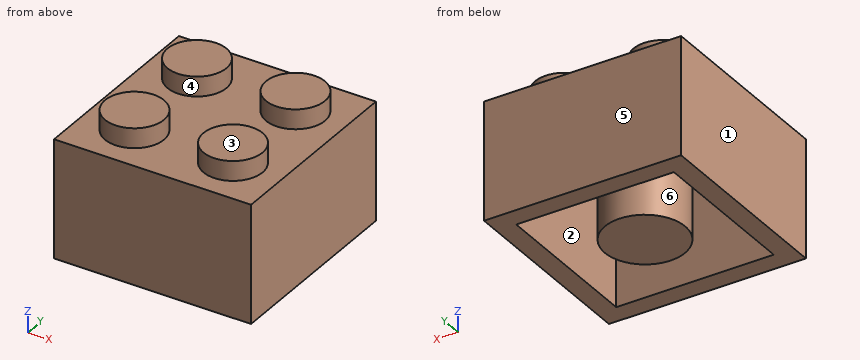
from build123d import *

# Parameters (mm, degrees)
F0_W     = 16
F0_H     = 16
F1_DEPTH = 9.6
F2_W     = 12.8
F2_H     = 12.8
F2_R     = 3.2565
F3_DEPTH = 8
F4_R     = 2.4
F5_DEPTH = 1.6
F6_R     = 1.2
F7_DEPTH = 1.6


with BuildPart() as f1:
    # F0 (on Top) → F1 (new body)
    with BuildSketch(Plane.XY):
        Rectangle(F0_W, F0_H)
    extrude(amount=F1_DEPTH)

    # F2 (on face) → F3 (cut)
    with BuildSketch(Plane(origin=(0, 0, 0), x_dir=(1, 0, 0), z_dir=(0, 0, -1))):
        Rectangle(F2_W, F2_H)
        Circle(F2_R, mode=Mode.SUBTRACT)
    extrude(amount=-F3_DEPTH, mode=Mode.SUBTRACT)

    # F4 (on face) → F5 (join)
    with BuildSketch(Plane.XY.offset(9.6)):
        with Locations((-4, 4)):
            Circle(F4_R)
        with Locations((4, 4)):
            Circle(F4_R)
        with Locations((-4, -4)):
            Circle(F4_R)
        with Locations((4, -4)):
            Circle(F4_R)
    extrude(amount=F5_DEPTH)

    # F6 (on face) → F7 (cut)
    with BuildSketch(Plane(origin=(0, 0, 8), x_dir=(1, 0, 0), z_dir=(0, 0, -1))):
        with Locations((-4, -4)):
            Circle(F6_R)
        with Locations((4, -4)):
            Circle(F6_R)
        with Locations((-4, 4)):
            Circle(F6_R)
        with Locations((4, 4)):
            Circle(F6_R)
    extrude(amount=-F7_DEPTH, mode=Mode.SUBTRACT)


solid = f1.part
Here's how the part is built. I have some questions about the finished solid (model axes, mm). Face numbers are marked on the shaded views. A direction names the side the tool comes from. Round coordinates to 2 decimals unless told otherwise and drop trailing zeros. Loops run counter-clockwise (first coordinate to the right, second up) from the corner with the lowest first, then second, coordinate; pieces in that order, holes last. Notation, with made-up numbers: (87, 77.25) -> (122, 77.25) arc R18 cw to (122, 106.25) -> close; hole circle Ø11 at (69.5, 66). An arc over 180 degrees is marked (long way). Write each question's results on one line, items separated by ' | '.
(1) For the marked faces 4, 5 and 6, which set-ups out of +Z, -Z, +X, -X, +Y, -Y let a thin tool reach every point of the face, with its end or its side?
Worked answers:
face 4: +Z | face 5: +Z, -Z, +X, -X, +Y | face 6: -Z
(2) If I drill on L1, parallel to X at y = 4, z = 8.75; L2, parallel to X at y = 0, z = 4, over which ranges is the centre line in solid material (lowest first)?
Worked answers:
L1: -8 to -5.2, -2.8 to 2.8, 5.2 to 8 | L2: -8 to -6.4, -3.26 to 3.26, 6.4 to 8
(3) For P1, Ø3, axis at x = 2, y = -2, coming from the +Z side; P2, Ø1.2, axis at x = -4.5, y = -4, coming from the -Z side; P3, Ø2.5, axis at x = -3.5, y = 4.5, coming from the -Z side, each with a flat end and sliding along its axis, tell me the tip position at first contact or that it passes through.
Worked answers:
P1: z = 11.2 | P2: z = 9.6 | P3: z = 8
(4) If we section it at A-A, the plane z = 4.5: List the corners of the cut face in (x, y) for me.
Worked answers:
outline: (-8, -8) -> (8, -8) -> (8, 8) -> (-8, 8) -> close; circle Ø6.51 at (0, 0); hole (-6.4, -6.4) -> (6.4, -6.4) -> (6.4, 6.4) -> (-6.4, 6.4) -> close
(5) We'd pull the mould along X, two halves only. Please class the marked faces 1, 2 and 3: released by +X, released by -X, zero draft, split by the parting line, or undercut.
Worked answers:
face 1: released by -X | face 2: undercut | face 3: zero draft
(6) If we section it at B-B, the plane x = -4: List the corners of the cut face in (y, z) for me, then the cut area to 3 significant figures.
Worked answers:
outline: (-8, 0) -> (-6.4, 0) -> (-6.4, 8) -> (-5.2, 8) -> (-5.2, 9.6) -> (-2.8, 9.6) -> (-2.8, 8) -> (2.8, 8) -> (2.8, 9.6) -> (5.2, 9.6) -> (5.2, 8) -> (6.4, 8) -> (6.4, 0) -> (8, 0) -> (8, 9.6) -> (6.4, 9.6) -> (6.4, 11.2) -> (1.6, 11.2) -> (1.6, 9.6) -> (-1.6, 9.6) -> (-1.6, 11.2) -> (-6.4, 11.2) -> (-6.4, 9.6) -> (-8, 9.6) -> close | area: 58.9 mm2
(7) If we section it at D-D, the plane x = 0: List the corners of the cut face in (y, z) for me, then the cut area to 3 significant figures.
Worked answers:
outline: (-8, 0) -> (-6.4, 0) -> (-6.4, 8) -> (-3.26, 8) -> (-3.26, 0) -> (3.26, 0) -> (3.26, 8) -> (6.4, 8) -> (6.4, 0) -> (8, 0) -> (8, 9.6) -> (-8, 9.6) -> close | area: 103 mm2
